Input: part model. Units: mm. Frame: model coordinates. Round coordinates to 2 decimals unless told otherwise and drop trailing zeros. Loops run counter-clockwise (first coordinate to the right, second up) from the corner with the lowest first, then second, coordinate; pieces in that order, holes last. Notation, with made-up numbers: (32.5, -15) - (66.5, -15) arc R24 cw to (66.5, 16) - close; hole circle Ø2 at (46, 12). An arc over 180 degrees is marked (long way). Use CSV: the item, a comma, the result in double quotes. Start each with the question number.
1. Material intervals for probe 1 along X at (y, z) = (-0.4, -0.65); probe 2 along X at (y, z) = (-2.2, 0.1); probe 3 along Y at (x, z) = (3, 0.5), sorted ascending. Write a range as from..to.
2. Pin query (flat end, axial travel): P1, Ø1, axis at x = 2, y = 0, coming from the -Z side; P2, Ø2, axis at x = -3.5, y = -2, coming from the -Z side; P3, Ø1, axis at x = 4.5, y = 0, coming from the +Z side. Return the tip coordinate at first contact, or that it passes through.
3. Cut plane A-A (x = 5.5). Return loops of the section in (y, z).
```python
from build123d import *

# Parameters (mm, degrees)
FILLET2_R = 0.25
SKETCH4_R = 0.25


with BuildPart() as part:
    # Sketch1 → Revolve1 (revolve)
    with BuildSketch(Plane.XY):
        with BuildLine():
            Line((-3.5, 0), (3.5, 0))
            Line((3.5, 0), (3.5, 1.5))
            add(Edge.make_bspline(
                [(-3.5, 1.5), (0, 0.282452635), (3.5, 1.5)],
                knots=[0, 0, 0, 1, 1, 1], degree=2))
            Line((-3.5, 1.5), (-3.5, 0))
        make_face()
    revolve(axis=Axis((-3.5, 0, 0), (1, 0, 0)))

    # Fillet2
    fillet2_edges = [part.edges().sort_by_distance(p)[0] for p in [
        (3.5, -1.5, 0),
        (-3.5, -1.5, 0),
    ]]
    fillet(fillet2_edges, radius=FILLET2_R)

    # Sweep1: sweep along a path in Sketch3
    with BuildLine(Plane.XY) as sweep1_path:
        Line((3.5, 0), (5.75, 0))
        ThreePointArc((5.75, 0), (6.103553391, -0.146446609), (6.25, -0.5))
        Line((6.25, -0.5), (6.25, -3))
    # Sketch4 → Sweep1 (sweep)
    with BuildSketch(Plane(origin=(3.5, 0, 0), x_dir=(0, 0, -1), z_dir=(1, 0, 0))):
        Circle(SKETCH4_R)
    sweep1 = sweep(path=sweep1_path.line)

    # Mirror1: Sweep1 across plane
    add(sweep1.mirror(Plane(origin=(0, 0, 0), x_dir=(0, 0, 1), z_dir=(1, 0, 0))))


solid = part.part
```
Established:
1,probe 1,"x = -3.5..3.5"
1,probe 2,"x = -6.48..-6.02, 6.02..6.48"
1,probe 3,"y = -1.24..1.24"
2,P1,"stops at z = -1.2"
2,P2,"stops at z = -0.96"
2,P3,"stops at z = 0.25"
3,outline,"circle Ø0.5 at (0, 0)"
